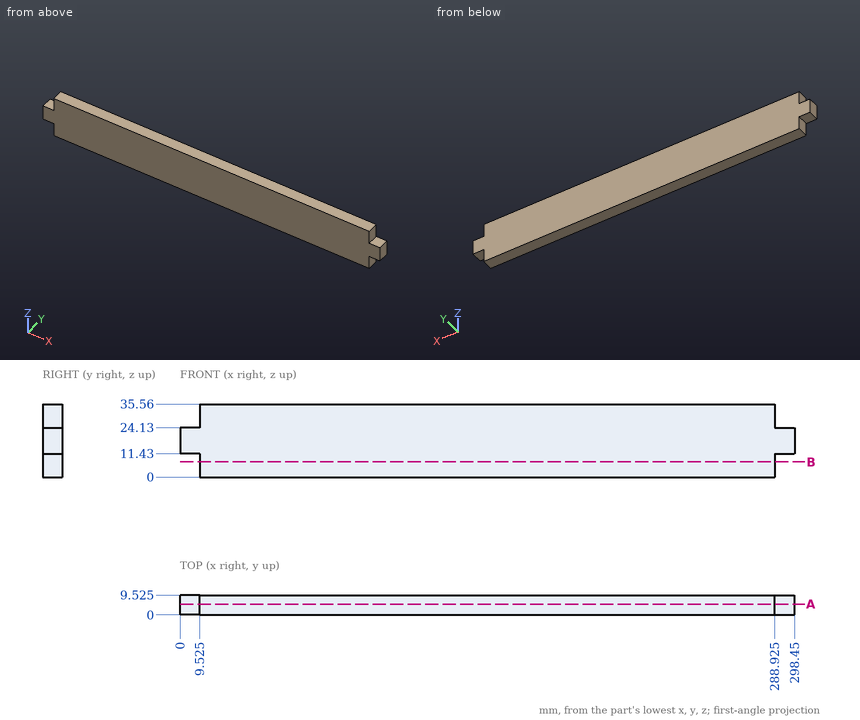
Answer from the drawing. Dimensions are ordinates in mm from the lowest x, y and z of the part. Give positions to 0.01 mm unless a question says otherwise; leave off trailing zeros. Write each loop counter-clockwise with the first axis right and the second up, starting at its lowest first coordinate (ties: lowest second). Pieces come first, ordered by that corner, then holes. Notation, with made-up numbers: (13, 53.25) - (69, 53.25) arc R10 cw to (69, 67.25) - close; hole circle Ø4 at (56, 24). An arc over 180 degrees is marked (long way). Answer in a Markdown table with one row per item. Add a question column.
Item 1: Section B-B, the plane z = 7.5 is taken. Write down the section's boundary in (x, y) (3 decimals).
Item 2: Find the intervals of material crossed by L1, parallel to X at y = 6.25, z = 4 (3 decimals), in increasing order.
Item 3: Section A-A, the plane y = 5.25 is taken. Write down the section's boundary in (x, z) (3 decimals), and give its area (3 significant figures).
Item 4: Flat-ended cylindrical pins translate along their axes: P1, Ø5, axis at x = 4, y = 4.5, coming from the -Z side; P2, Ø3, axis at y = 6, z = 4.5, coming from the -X side (3 decimals); P3, Ø1.5, axis at y = 5, z = 31, coming from the +X side (3 decimals). Find the tip coordinate at first contact, or state that the pin passes through.
Recorded:
| question | item | result |
|---|---|---|
| 1 | outline | (9.525, 0) - (288.925, 0) - (288.925, 9.525) - (9.525, 9.525) - close |
| 2 | L1 | x = 9.525 to 288.925 |
| 3 | outline | (0, 11.43) - (9.525, 11.43) - (9.525, 0) - (288.925, 0) - (288.925, 11.43) - (298.45, 11.43) - (298.45, 24.13) - (288.925, 24.13) - (288.925, 35.56) - (9.525, 35.56) - (9.525, 24.13) - (0, 24.13) - close |
| 3 | area | 10,200 mm2 |
| 4 | P1 | stops at z = 11.43 |
| 4 | P2 | stops at x = 9.525 |
| 4 | P3 | stops at x = 288.925 |
